```python
from build123d import *

# Parameters (mm, degrees)
F0_R     = 11.176
F1_DEPTH = 6.35


with BuildPart() as f1:
    # F0 (on Front) → F1 (new body)
    with BuildSketch(Plane.XZ):
        with BuildLine():
            ThreePointArc((12.7517006508, 23.4892014836), (15.490274076, 28.359134381), (16.4396849361, 33.8650085032))
            ThreePointArc((16.4396849361, 33.8650085032), (-5.7959286408, 49.2491058764), (-12.3528926478, 23.0174611293))
            ThreePointArc((-12.3528926478, 23.0174611293), (-12.2109180853, 22.8621908621), (-12.0712241226, 22.7048656287))
            ThreePointArc((-12.0712241226, 22.7048656287), (-0.3017671927, 17.4280934228), (11.6534468913, 22.2693016964))
            ThreePointArc((11.6534468913, 22.2693016964), (12.1852012792, 22.8948917308), (12.7517006508, 23.4892014836))
        make_face()
        with BuildLine():
            ThreePointArc((-12.0712241226, 22.7048656287), (-12.2109180853, 22.8621908621), (-12.3528926478, 23.0174611293))
            ThreePointArc((-12.3528926478, 23.0174611293), (-12.2130585437, 22.8602621723), (-12.0712241226, 22.7048656287))
        make_face()
        with BuildLine():
            ThreePointArc((-12.0712241226, 22.7048656287), (-12.2130585437, 22.8602621723), (-12.3528926478, 23.0174611293))
            ThreePointArc((-12.3528926478, 23.0174611293), (-35.2568762282, 20.6796890684), (-26.7180955248, -0.7013040367))
            ThreePointArc((-26.7180955248, -0.7013040367), (-25.9110393194, -0.8518354275), (-25.1125044392, -1.0424697987))
            ThreePointArc((-25.1125044392, -1.0424697987), (-13.5329586121, 2.2669935247), (-8.5036933239, 13.2097957122))
            ThreePointArc((-8.5036933239, 13.2097957122), (-9.4250093039, 18.2813740839), (-12.0712241226, 22.7048656287))
        make_face()
        with BuildLine():
            ThreePointArc((37.321032921, 13.2471223209), (28.4497702153, 26.5564449349), (12.7517006508, 23.4892014836))
            ThreePointArc((12.7517006508, 23.4892014836), (12.2178085396, 22.8655360028), (11.6534468913, 22.2693016964))
            ThreePointArc((11.6534468913, 22.2693016964), (10.5710761807, 5.7719047545), (25.6986024853, -0.8984460694))
            ThreePointArc((25.6986024853, -0.8984460694), (25.9040970502, -0.8533121295), (26.1101523925, -0.8108117214))
            ThreePointArc((26.1101523925, -0.8108117214), (34.1751435518, 4.2567197748), (37.321032921, 13.2471223209))
        make_face()
        with BuildLine():
            ThreePointArc((11.6534468913, 22.2693016964), (12.2178085396, 22.8655360028), (12.7517006508, 23.4892014836))
            ThreePointArc((12.7517006508, 23.4892014836), (12.1852012792, 22.8948917308), (11.6534468913, 22.2693016964))
        make_face()
        with BuildLine():
            ThreePointArc((-25.1125044392, -1.0424697987), (-25.9201584954, -0.8947520073), (-26.7180955248, -0.7013040367))
            ThreePointArc((-26.7180955248, -0.7013040367), (-43.4081977491, -25.41837957), (-13.7572597447, -22.2066494078))
            ThreePointArc((-13.7572597447, -22.2066494078), (-13.6937790301, -22.0060606965), (-13.6273783627, -21.8064195594))
            ThreePointArc((-13.6273783627, -21.8064195594), (-13.0740993856, -19.3973230871), (-12.8882727271, -16.9325042516))
            ThreePointArc((-12.8882727271, -16.9325042516), (-16.2979161501, -6.9084701851), (-25.1125044392, -1.0424697987))
        make_face()
        with BuildLine():
            ThreePointArc((-25.1125044392, -1.0424697987), (-25.9110393194, -0.8518354275), (-26.7180955248, -0.7013040367))
            ThreePointArc((-26.7180955248, -0.7013040367), (-25.9201584954, -0.8947520073), (-25.1125044392, -1.0424697987))
        make_face()
        with BuildLine():
            ThreePointArc((-13.6273783627, -21.8064195594), (-13.6937790301, -22.0060606965), (-13.7572597447, -22.2066494078))
            ThreePointArc((-13.7572597447, -22.2066494078), (-13.6910385066, -22.0069500429), (-13.6273783627, -21.8064195594))
        make_face()
        with BuildLine():
            ThreePointArc((-13.6273783627, -21.8064195594), (-13.6910385066, -22.0069500429), (-13.7572597447, -22.2066494078))
            ThreePointArc((-13.7572597447, -22.2066494078), (-2.127588621, -40.7153049273), (14.44099559, -26.4569180331))
            ThreePointArc((14.44099559, -26.4569180331), (14.3218531968, -24.6071235917), (13.966394874, -22.7878974469))
            ThreePointArc((13.966394874, -22.7878974469), (13.6932307798, -22.0137005753), (13.459057548, -21.2268318977))
            ThreePointArc((13.459057548, -21.2268318977), (-0.2869219447, -12.0407728951), (-13.6273783627, -21.8064195594))
        make_face()
        with BuildLine():
            ThreePointArc((26.1101523925, -0.8108117214), (25.9046971154, -0.8561301656), (25.6986024853, -0.8984460694))
            ThreePointArc((25.6986024853, -0.8984460694), (15.24405524, -8.4527086566), (13.459057548, -21.2268318977))
            ThreePointArc((13.459057548, -21.2268318977), (13.7349572161, -22.0001397234), (13.966394874, -22.7878974469))
            ThreePointArc((13.966394874, -22.7878974469), (32.3048678413, -33.100412174), (45.7676425992, -16.9325042516))
            ThreePointArc((45.7676425992, -16.9325042516), (39.7530124822, -4.2210341235), (26.1101523925, -0.8108117214))
        make_face()
        with BuildLine():
            ThreePointArc((26.1101523925, -0.8108117214), (25.9040970502, -0.8533121295), (25.6986024853, -0.8984460694))
            ThreePointArc((25.6986024853, -0.8984460694), (25.9046971154, -0.8561301656), (26.1101523925, -0.8108117214))
        make_face()
        with BuildLine():
            ThreePointArc((13.966394874, -22.7878974469), (13.7349572161, -22.0001397234), (13.459057548, -21.2268318977))
            ThreePointArc((13.459057548, -21.2268318977), (13.6932307798, -22.0137005753), (13.966394874, -22.7878974469))
        make_face()
        with BuildLine():
            ThreePointArc((11.6534468913, 22.2693016964), (-0.3017671927, 17.4280934228), (-12.0712241226, 22.7048656287))
            ThreePointArc((-12.0712241226, 22.7048656287), (-9.4250093039, 18.2813740839), (-8.5036933239, 13.2097957122))
            ThreePointArc((-8.5036933239, 13.2097957122), (-13.5329586121, 2.2669935247), (-25.1125044392, -1.0424697987))
            ThreePointArc((-25.1125044392, -1.0424697987), (-16.2979161501, -6.9084701851), (-12.8882727271, -16.9325042516))
            ThreePointArc((-12.8882727271, -16.9325042516), (-13.0740993856, -19.3973230871), (-13.6273783627, -21.8064195594))
            ThreePointArc((-13.6273783627, -21.8064195594), (-0.2869219447, -12.0407728951), (13.459057548, -21.2268318977))
            ThreePointArc((13.459057548, -21.2268318977), (15.24405524, -8.4527086566), (25.6986024853, -0.8984460694))
            ThreePointArc((25.6986024853, -0.8984460694), (10.5710761807, 5.7719047545), (11.6534468913, 22.2693016964))
        make_face()
        Circle(F0_R, mode=Mode.SUBTRACT)
    extrude(amount=F1_DEPTH)


solid = f1.part
```
The listing builds one solid part. Answer for the finished solid, in the listing's coordinates (mm). Round coordinates to 2 decimals unless told otherwise and drop trailing zeros. Loops run counter-clockwise (first coordinate to the right, second up) from the corner with the lowest first, then second, coordinate; pieces in that order, holes last.
Q1. Given pin 1 Ø2 at (x, y) = (-4.5, -2) entering from -Z; pin 2 Ø12 at (x, z) = (3.5, 6) entering from +Y; pin 3 Ø1.5 at (y, z) = (-4.5, 39) entering from -X; pin 4 Ø2 at (x, z) = (-18.5, 36.5) entering from +Y, each flat-ended and moving along its own axis, determine where each tip first touches the part or whether it passes through.
Q2. For a pull along Z with two mould halves and no side action, classify faces 1 (the face through (-8.87, -3.13, -6.8)), 2 (the face through (-11, 0, 5)) as released by +Z, released by -Z, zero draft, split by the parting line, or undercut.
Q3. Section A-A, the plane x = 0 is taken. Determine the outline of the cut face in (y, z).
Q4. Section B-B, the plane z = 26.5 is taken. Determine the outline of the cut face in (x, y), then the cut area to 3 significant figures.
Q5. Find the intervals of material crossed by line 1 (Z direction, x = 0, y = -4.5); line 2 (X direction, y = -3.25, z = 34); line 3 (Z direction, x = 9.5, y = -2), in increasing order.
Q6. Section D-D, the plane x = 27.5 is taken. Determine the outline of the cut face in (y, z).
Q7. Section C-C, the plane y = -4.5 is taken. Determine the outline of the cut face in (x, z) (1 decimal), then the cut area to 3 significant figures.
Completed:
1. pin 1: stops at z = -40.44
1. pin 2: stops at y = 0
1. pin 3: stops at x = -15.84
1. pin 4: passes through
2. face 1: undercut
2. face 2: zero draft
3. outline: (-6.35, -40.88) - (0, -40.88) - (0, -11.18) - (-6.35, -11.18) - close; (-6.35, 11.18) - (0, 11.18) - (0, 50.3) - (-6.35, 50.3) - close
4. outline: (-28.52, -6.35) - (-17.33, -6.35) - (-17.33, 0) - (-28.52, 0) - close; (-14.7, -6.35) - (14.7, -6.35) - (14.7, 0) - (-14.7, 0) - close; (17.22, -6.35) - (28.58, -6.35) - (28.58, 0) - (17.22, 0) - close
4. area: 330 mm2
5. line 1: z = -40.88 to -11.18, 11.18 to 50.3
5. line 2: x = -16.44 to 16.44
5. line 3: z = -37.32 to -5.89, 5.89 to 47.28
6. outline: (-6.35, -33.27) - (0, -33.27) - (0, -0.59) - (-6.35, -0.59) - close; (-6.35, -0.42) - (0, -0.42) - (0, 26.91) - (-6.35, 26.91) - close
7. outline: (-26.7, -0.7) arc R16.4 ccw (long way) to (-13.8, -22.2) arc R14.4 ccw (long way) to (14, -22.8) arc R16.4 ccw (long way) to (26.1, -0.8) arc R14.4 ccw (long way) to (12.8, 23.5) arc R16.4 ccw (long way) to (-12.4, 23) arc R14.4 ccw (long way) to start; hole circle Ø22.4 at (0, 0)
7. area: 4,980 mm2
